```python
from build123d import *

# Parameters (mm, degrees)
SKETCH_1_W      = 45
SKETCH_1_H      = 100
EXTRUDE_1_DEPTH = 4
SKETCH_2_W      = 40
SKETCH_2_H      = 95
EXTRUDE_2_DEPTH = 4
FILLET_1_R      = 5


with BuildPart() as part:
    # 草圖1 → 填料-伸長1 (new body)
    with BuildSketch(Plane.XY):
        Rectangle(SKETCH_1_W, SKETCH_1_H)
    extrude(amount=EXTRUDE_1_DEPTH)

    # 草圖2 → 填料-伸長2 (add)
    with BuildSketch(Plane.XY.offset(4)):
        Rectangle(SKETCH_2_W, SKETCH_2_H)
    extrude(amount=EXTRUDE_2_DEPTH)

    # 圓角1
    fillet_1_edges = [part.edges().sort_by_distance(p)[0] for p in [
        (20, -47.5, 6),
        (20, 47.5, 6),
        (-20, 47.5, 6),
        (-20, -47.5, 6),
        (22.5, -50, 2),
        (-22.5, -50, 2),
        (-22.5, 50, 2),
        (22.5, 50, 2),
    ]]
    fillet(fillet_1_edges, radius=FILLET_1_R)


solid = part.part
```
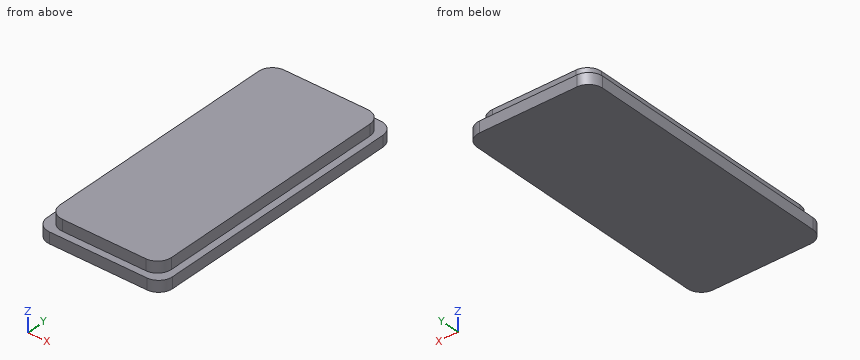
Geometry: final body of the model. Coordinates: model frame, mm. Coordinates: 2 decimals unless noted, no trailing zeros. Write each loop counter-clockwise with the first axis right and the second up, starting at its lowest first coordinate (ties: lowest second). Pieces come first, ordered by that corner, then holes. Notation, with made-up numbers: M 52.25,-5.75 L 96.25,-5.75 A26 ccw 96.25,16.25 Z; hole C 88,18.25 d10. An arc over 180 degrees is marked long. Use CSV: the item, a comma, the result in double quotes. Start each with the question number.
1. Ray query, probe 1 along X at (y, z) = (-29, 7.75); probe 2 along Y at (x, z) = (2, 6.5); probe 3 along Y at (x, z) = (19.5, 5.25). Return the intervals inside material, ascending.
2. Cut plane A-A on y = -30. Return the cut outline in (x, z), plus the area to 3 significant figures.
3. First-contact query: P1, Ø2, axis at x = -5, z = 7, coming from the +Y side; P2, Ø2, axis at y = -3, z = 5.5, coming from the -X side; P3, Ø2, axis at y = -5, z = 5.5, coming from the +X side. Flat tips, straight axial feed; report the tip coordinate or a pass-through.
4. Cut plane B-B on z = 6.75. Return the cut outline in (x, y).
Entries:
1,probe 1,"-20 to 20"
1,probe 2,"-47.5 to 47.5"
1,probe 3,"-44.68 to 44.68"
2,outline,"M -22.5,0 L 22.5,0 L 22.5,4 L 20,4 L 20,8 L -20,8 L -20,4 L -22.5,4 Z"
2,area,"340 mm²"
3,P1,"y = 47.5"
3,P2,"x = -20"
3,P3,"x = 20"
4,outline,"M -20,-42.5 A5 ccw -15,-47.5 L 15,-47.5 A5 ccw 20,-42.5 L 20,42.5 A5 ccw 15,47.5 L -15,47.5 A5 ccw -20,42.5 Z"
